The listing builds one solid part. Answer for the finished solid, in the listing's coordinates (mm). A direction names the side the tool comes from. Give positions to 0.01 mm unless a question says otherwise; leave off trailing zeros. Write each loop counter-clockwise with the first axis right and the second up, starting at its lowest first coordinate (ties: lowest second). Pieces come first, ordered by that corner, then holes. Notation, with made-up numbers: M -10,28.5 L 27,28.5 A28 cw 27,55.5 Z; hole C 46,23 d1. An arc over 180 degrees is marked long. Answer as a JSON object with one key per item and string values.
```python
from build123d import *

# Parameters (mm, degrees)
BOSS_EXTRUDE1_DEPTH = 10
SKETCH2_R           = 2.625
CUT_EXTRUDE1_DEPTH  = 100.49874371
SKETCH3_R           = 12.2
CUT_EXTRUDE2_DEPTH  = 20
CUT_EXTRUDE3_DEPTH  = 4


with BuildPart() as part:
    # Sketch1 → Boss-Extrude1 (new body)
    with BuildSketch(Plane.XY):
        with BuildLine():
            Line((0, 70), (0, 0))
            Line((0, 0), (-70, 0))
            ThreePointArc((-70, 0), (-49.497474683, 49.497474683), (0, 70))
        make_face()
    extrude(amount=BOSS_EXTRUDE1_DEPTH)

    # Sketch2 → Cut-Extrude1 (cut, through all)
    with BuildSketch(Plane.XY):
        with Locations((-7.76457135, 28.97777479)):
            Circle(SKETCH2_R)
        with Locations((-21.213203434, 21.213203438)):
            Circle(SKETCH2_R)
        with Locations((-28.977774788, 7.764571356)):
            Circle(SKETCH2_R)
    extrude(amount=CUT_EXTRUDE1_DEPTH, mode=Mode.SUBTRACT)

    # Sketch3 → Cut-Extrude2 (cut)
    with BuildSketch(Plane.XY):
        Circle(SKETCH3_R)
    extrude(amount=CUT_EXTRUDE2_DEPTH, mode=Mode.SUBTRACT)

    # Sketch4 → Cut-Extrude3 (cut)
    with BuildSketch(Plane.XY):
        Polygon((-20.139437084, 31.464597344), (-35.69578627, 47.02094653), (-47.009494769, 35.707238031), (-31.453145583, 20.150888845), align=None)
        Polygon((-1.708965461, 37.318859162), (-17.163778681, 33.17775444), (-22.857797674, 54.428122618), (-7.402984453, 58.56922734), align=None)
        Polygon((-33.173562805, 17.179422078), (-54.423930983, 22.87344107), (-58.565035705, 7.418627849), (-37.314667526, 1.724608857), align=None)
    extrude(amount=CUT_EXTRUDE3_DEPTH, mode=Mode.SUBTRACT)


solid = part.part
```
1. A cutting plane is placed at A-A, the plane y = 9. Give the vertices of the cut face in (x, z).
Verdict:
{"outline": "M -69.42,0 L -58.14,0 L -58.14,4 L -35.37,4 L -35.37,0 L -31.29,0 L -31.29,10 L -69.42,10 Z; M -26.66,0 L -8.24,0 L -8.24,10 L -26.66,10 Z"}
2. A cutting plane is placed at D-D, the plane y = 16. Give the vertices of the cut face in (x, z), plus the area to 3 significant figures.
Verdict:
{"outline": "M -68.15,0 L -56.27,0 L -56.27,4 L -33.49,4 L -33.49,0 L 0,0 L 0,10 L -68.15,10 Z", "area": "590 mm2"}
3. Flat-ended cylindrical pins translate along their axes: pin 1 (3 mm diameter, centred on x = -13, z = 6, fed in from +Y); pin 2 (1.5 mm diameter, centred on y = 7, z = 8, fed in from +X); pin 3 (6 mm diameter, centred on x = -49, z = 5.5, fed in from +Y). Find the tip coordinate at first contact, or state that the pin passes through.
Verdict:
{"pin 1": "stops at y = 69.05", "pin 2": "stops at x = -9.42", "pin 3": "stops at y = 52.76"}
4. The mould has two halves that part along X. Classify faces 3 (the flat face through (-43.65, 19.987, 1.972)), 4 (the flat face through (-41, 0, 5)), 5 (the flat face through (0, 42, 5)): released by +X, released by -X, zero draft, split by the parting line, or undercut.
Verdict:
{"face 3": "undercut", "face 4": "zero draft", "face 5": "released by +X"}
5. Consider line 1 along Y through (x, z) = (-38, 3.25); line 2 along Y through (x, z) = (-45.5, 3.5); line 3 along Y through (x, z) = (-20.5, 7). Determine where each line is inside the solid, lowest interval first.
Verdict:
{"line 1": "y = 0 to 1.91, 18.47 to 26.7, 44.72 to 58.79", "line 2": "y = 0 to 3.92, 20.48 to 34.2, 37.22 to 53.2", "line 3": "y = 0 to 18.69, 23.74 to 66.93"}
6. For faces 1 (the flat face through (-27, 28, 10)), 2 (the flat face through (-41.273, 41.443, 1.972)), determine the directions among +Z, -Z, +X, -X, +Y, -Y from which every point of the face is accessible in a straight line to the end or side of a thin tool.
Verdict:
{"face 1": "+Z, +X, -X, +Y, -Y", "face 2": "-Z"}
7. A cutting plane is placed at B-B, the plane x = -57.5. Give the vertices of the cut face in (y, z).
Verdict:
{"outline": "M 0,0 L 7.13,0 L 7.13,4 L 11.39,4 L 11.39,0 L 39.92,0 L 39.92,10 L 0,10 Z"}
8. A cutting plane is placed at C-C, the plane z = 3. Count the separate pieces of the cut face and the enclosed holes in it, plus the area to 3 significant figures.
Verdict:
{"separate pieces": "1", "enclosed holes": "6", "area": "2,610 mm2"}
